Source: CAD feature listing. Evaluate the final solid. Frame: model axes, mm. A direction names the side the tool comes from. Round coordinates to 2 decimals unless told otherwise and drop trailing zeros. Loops run counter-clockwise (first coordinate to the right, second up) from the corner with the lowest first, then second, coordinate; pieces in that order, holes last. Notation, with made-up numbers: (-27, 22) -> (18, 22) arc R15 ccw to (18, 43) -> close; hole circle Ø9 at (14.25, 60). An arc over 180 degrees is marked (long way). Put each result on its own line as item: value. Start each with the question number.
1. Contact query for a flat-ended pin moving along its axis: pin 1 (2 mm diameter, centred on y = -2, z = 1, fed in from -X). Output: stop coordinate, or through.
2. Material intervals for L1, parallel to Z at x = 1.5, y = -4.5; L2, parallel to Y at x = 1.4, z = 3.5; L3, parallel to X at y = -2.5, z = 3, sorted ascending.
3. Cut plane B-B (x = 1.5). Return the cut outline in (y, z).
4. Cut plane C-C (y = -19.75). Return the cut outline in (x, z), then the cut area to 3 significant figures.
5. Draft query along Z for faces 3 (the cylindrical face through (1.521, -21.098, 6.098)), 4 (the flat face through (0.8, 0.546, 2.7)), 5 (the cylindrical face through (1.521, -20.285, 2.808)), 6 (the cylindrical face through (1.085, -2.905, 2.702)). Return one class per face: pulls with the +Z half, pulls with the -Z half, needs draft (parallel to the pull), parting line crosses it, or undercut.
6. Cut plane D-D (z = 1). Return the cut outline in (x, y), then the cut area to 3 significant figures.
7. Set-up query: faces 1 (the flat face through (2, -6.454, 4)), 2 (the flat face through (0, -11, 3)). Return all of +Z, -Z, +X, -X, +Y, -Y with unobstructed straight access to the full face (end or side cutting, diameter ignored); none if empty.
8. Cut plane A-A (z = 3.5). Return the cut outline in (x, y), then the cut area to 3 significant figures.
```python
from build123d import *

# Parameters (mm, degrees)
SKETCH_1_W          = 3
SKETCH_1_H          = 22.5
EXTRUDE_1_DEPTH     = 7
SKETCH_4_R          = 1.5
CUT_EXTRUDE_2_DEPTH = 24.237188714
FILLET_1_R          = 3
SKETCH_3_R          = 0.9
CUT_EXTRUDE_4_DEPTH = 7


with BuildPart() as part:
    # 草图1 → 凸台-拉伸1 (new body)
    with BuildSketch(Plane.XY):
        with Locations((1.5, -10.703745451)):
            Rectangle(SKETCH_1_W, SKETCH_1_H)
    extrude(amount=EXTRUDE_1_DEPTH)

    # 草图4 → 切除-拉伸2 (cut, through all)
    with BuildSketch(Plane(origin=(3, 0, 0), x_dir=(0, 0, -1), z_dir=(1, 0, 0))):
        with Locations((-3.5, -18.953745451)):
            Circle(SKETCH_4_R)
    extrude(amount=-CUT_EXTRUDE_2_DEPTH, mode=Mode.SUBTRACT)

    # 圆角1
    fillet_1_edges = [part.edges().sort_by_distance(p)[0] for p in [
        (1.5, -21.953745451, 7),
        (1.5, -21.953745451, 0),
    ]]
    fillet(fillet_1_edges, radius=FILLET_1_R)

    # 草图3 → 切除-拉伸4 (cut)
    with BuildSketch(Plane(origin=(0, 0.546254549, 0), x_dir=(1, 0, 0), z_dir=(0, 1, 0))):
        with Locations(Location((1.5, -3.5, 0), (0, 0, 180))):
            Circle(SKETCH_3_R)
    extrude(amount=-CUT_EXTRUDE_4_DEPTH, mode=Mode.SUBTRACT)


solid = part.part
```
Solution:
1. pin 1: stops at x = 0
2. L1: z = 0 to 2.6, 4.4 to 7
2. L2: y = -21.95 to -20.45, -17.45 to -6.45
2. L3: x = 0 to 0.75, 2.25 to 3
3. outline: (-21.95, 3) arc R3 ccw to (-18.95, 0) -> (0.55, 0) -> (0.55, 2.6) -> (-6.45, 2.6) -> (-6.45, 4.4) -> (0.55, 4.4) -> (0.55, 7) -> (-18.95, 7) arc R3 ccw to (-21.95, 4) -> close; hole circle Ø3 at (-18.95, 3.5)
4. outline: (0, 0.11) -> (3, 0.11) -> (3, 2.23) -> (0, 2.23) -> close; (0, 4.77) -> (3, 4.77) -> (3, 6.89) -> (0, 6.89) -> close
4. area: 12.7 mm^2
5. face 3: pulls with the +Z half
5. face 4: needs draft
5. face 5: undercut
5. face 6: undercut
6. outline: (0, -21.19) -> (3, -21.19) -> (3, 0.55) -> (0, 0.55) -> close
6. area: 65.2 mm^2
7. face 1: +Y
7. face 2: +Z, -Z, -X, +Y, -Y
8. outline: (0, -21.95) -> (3, -21.95) -> (3, -20.45) -> (0, -20.45) -> close; (0, -17.45) -> (3, -17.45) -> (3, 0.55) -> (2.4, 0.55) -> (2.4, -6.45) -> (0.6, -6.45) -> (0.6, 0.55) -> (0, 0.55) -> close
8. area: 45.9 mm^2
